from build123d import *

# Parameters (mm, degrees)
SKETCH1_R         = 4
BUMPER_LINK_DEPTH = 1


with BuildPart() as part:
    # Sketch1 → Bumper link (new body)
    with BuildSketch(Plane.XY):
        with BuildLine():
            Line((-12.339935794, -62.372114787), (-12.339935794, -64.125193558))
            ThreePointArc((-12.339935794, -64.125193558), (-11.942206179, -65.142543055), (-10.959935794, -65.620385853))
            Line((-10.959935794, -65.620385853), (10.959935794, -67.379614147))
            ThreePointArc((10.959935794, -67.379614147), (12.097285292, -66.986692236), (12.579935794, -65.884421852))
            Line((12.579935794, -65.884421852), (12.579935794, -64.13134308))
            ThreePointArc((12.579935794, -64.13134308), (13.061403486, -63.030165558), (14.196725042, -62.635896568))
            Line((14.196725042, -62.635896568), (52.610702507, -65.635896568))
            ThreePointArc((52.610702507, -65.635896568), (56.395107696, -64.321666601), (58, -60.65107486))
            Line((58, -60.65107486), (58, 37.364103432))
            ThreePointArc((58, 37.364103432), (56.535533906, 40.899637338), (53, 42.364103432))
            Line((53, 42.364103432), (47, 42.364103432))
            ThreePointArc((47, 42.364103432), (45.585786438, 42.94988987), (45, 44.364103432))
            Line((45, 44.364103432), (45, 54.449696626))
            ThreePointArc((45, 54.449696626), (43.937003937, 57.531903627), (41.2, 59.303561066))
            Line((41.2, 59.303561066), (-22.203206715, 74.978462786))
            ThreePointArc((-22.203206715, 74.978462786), (-27.378610186, 74.877873729), (-31.810346538, 72.203059315))
            Line((-31.810346538, 72.203059315), (-51.696396663, 51.528677297))
            ThreePointArc((-51.696396663, 51.528677297), (-54.153116802, 47.167307088), (-54.188361237, 42.161732018))
            Line((-54.188361237, 42.161732018), (-33.67267763, -39.569202441))
            ThreePointArc((-33.67267763, -39.569202441), (-26.339013672, -52.913431655), (-13.39876573, -60.938458979))
            ThreePointArc((-13.39876573, -60.938458979), (-12.633338286, -61.480979302), (-12.339935794, -62.372114787))
        make_face()
        with Locations((0, -57.5)):
            Circle(SKETCH1_R, mode=Mode.SUBTRACT)
        with Locations((-38.475009866, 42.730827465)):
            Circle(SKETCH1_R, mode=Mode.SUBTRACT)
        with Locations((38.475009866, 42.730827465)):
            Circle(SKETCH1_R, mode=Mode.SUBTRACT)
        with BuildLine():
            Line((32, 30.368569278), (32, -30.368569278))
            ThreePointArc((32, -30.368569278), (30.906926144, -34.914629844), (27.866666667, -38.466854419))
            ThreePointArc((27.866666667, -38.466854419), (9.287328638, -46.583210782), (-10.984071313, -46.212554327))
            ThreePointArc((-10.984071313, -46.212554327), (-15.698093899, -43.598992826), (-18.370739643, -38.918215391))
            Line((-18.370739643, -38.918215391), (-34.572943336, 25.628561282))
            ThreePointArc((-34.572943336, 25.628561282), (-34.427736148, 31.016661832), (-31.506862657, 35.546696127))
            ThreePointArc((-31.506862657, 35.546696127), (-2.333364057, 47.442653933), (27.866666667, 38.466854419))
            ThreePointArc((27.866666667, 38.466854419), (30.906926144, 34.914629844), (32, 30.368569278))
        make_face(mode=Mode.SUBTRACT)
    extrude(amount=BUMPER_LINK_DEPTH)


solid = part.part
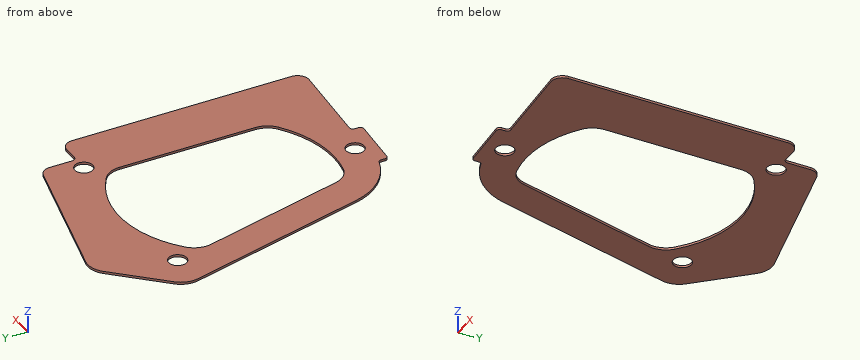
Check sheet for the modelled part. Datum: model origin and axes. Units: mm. Round coordinates to 2 decimals unless told otherwise and drop trailing zeros. Order: outer loops, then holes, each group sorted by start corner. A loop starts at its lowest first (then second) coordinate and runs counter-clockwise, first axis right, second up. Notation, with made-up numbers: M 62.25,1 L 112.25,1 A25 ccw 112.25,18 Z; hole C 45,-15 d9. An arc over 180 degrees is marked long. One line per item, written item: value. Start each with the question number.
1. Section check B-B on z = 0.2. Give the number of separate pieces and of enclosed holes in the cut face, and give its area (3 significant figures).
2. Section check A-A on x = -28. Enter the section's corners in (y, z), and give its area (3 significant figures).
3. Gauge pin test, flat ends, axial feed: P1, Ø7, axis at x = -38.48, y = 42.73, coming from the +Z side; P2, Ø0.5, axis at x = 51, z = 0.5, coming from the +Y side; P3, Ø0.5, axis at y = -64.5, z = 0.5, coming from the +X side. Record the tip position at first contact, or that the pin passes through.
4. Section check D-D on x = 0. Enter the section's corners in (y, z), and give its area (3 significant figures).
5. Section check C-C on y = -17. Enter the section's corners in (x, z).
6. Scan lines: line 1 along Y through (x, z) = (0, 0.7); line 2 along Y through (x, z) = (-0.5, 0.8); line 3 along X through (y, z) = (-43, 0.5). Record each from-to range of solid material in increasing order.
Results found:
1. separate pieces: 1
1. enclosed holes: 4
1. area: 7,430 mm^2
2. outline: M -51.01,0 L -0.56,0 L -0.56,1 L -51.01,1 Z; M 38.37,0 L 74.68,0 L 74.68,1 L 38.37,1 Z
2. area: 86.8 mm^2
3. P1: through
3. P2: y = 42.36
3. P3: x = 56.47
4. outline: M -66.5,0 L -61.5,0 L -61.5,1 L -66.5,1 Z; M -53.5,0 L -47.5,0 L -47.5,1 L -53.5,1 Z; M 47.5,0 L 69.49,0 L 69.49,1 L 47.5,1 Z
4. area: 33.0 mm^2
5. outline: M -39.34,0 L -23.87,0 L -23.87,1 L -39.34,1 Z; M 32,0 L 58,0 L 58,1 L 32,1 Z
6. line 1: -66.5 to -61.5, -53.5 to -47.5, 47.5 to 69.49
6. line 2: -66.46 to -61.47, -53.53 to -47.5, 47.5 to 69.61
6. line 3: -32.59 to -16.26, 20.18 to 58
